Check sheet for the drawn part. Datum: minimum x, y, z corner. Units: mm. A direction names the side the tool comes from. Round coordinates to 2 decimals unless told otherwise and drop trailing zeros. Write each loop counter-clockwise with the first axis right and the second up, starting at its lowest first coordinate (ties: lowest second). Pieces come first, ordered by that corner, then holes. Notation, with made-up numbers: (-11, -27.5) - (2, -27.5) arc R21 ccw to (2, 5.5) - close; hole circle Ø1 at (-35.5, -16). An arc over 180 degrees is marked (long way). Return JSON: item names as keys, results as strings. Group by question number.
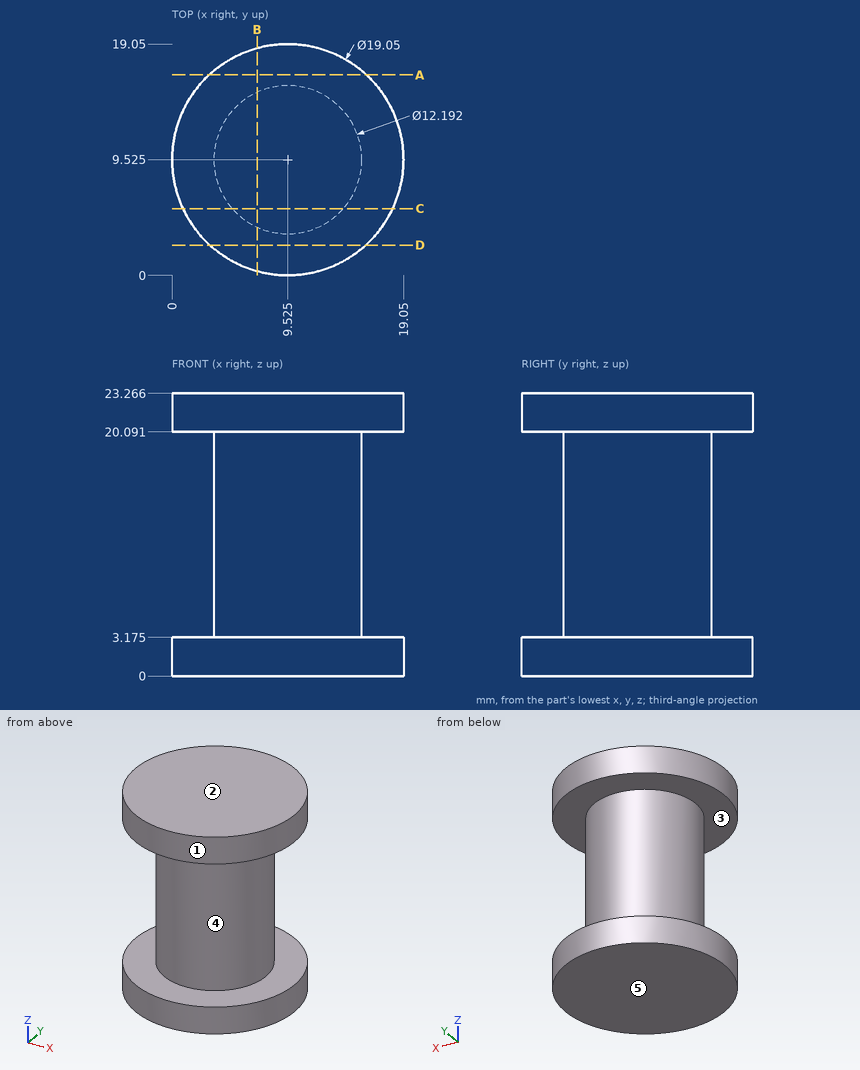
1. Mould release check, pull along Z, two halves, no side actions. Record for the marked faces 1, 2 and 3: pulls with the +Z half, pulls with the -Z half, needs draft (parallel to the pull), parting line crosses it, or undercut.
2. Material ranges on line 1 along Z through (x, y) = (3.5, 11.25) (1 decimal); line 2 along X through (y, z) = (9.75, 9.5); line 3 along Y through (x, z) = (5.25, 15.5), recorded low to high.
3. Section check B-B (x = 7). Enter the section's corners in (y, z) (1 decimal), and give its area (3 significant figures).
4. Tool access check on the marked faces 4 and 5. Record the directions out of +Z, -Z, +X, -X, +Y, -Y that give a thin tool (end or side, any length) a straight path to the whole face; none if there is none.
5. Section check C-C (y = 5.5). Enter the section's corners in (x, z) (1 decimal).
6. Section check D-D (y = 2.5). Enter the section's corners in (x, z) (1 decimal).
7. Section check A-A (y = 16.5). Enter the section's corners in (x, z) (1 decimal).
8. Depth check by flat-ended pin: pin 1 Ø2 at (y, z) = (6.5, 15) entering from -X (1 decimal); pin 2 Ø10 at (y, z) = (17, 19.5) entering from -X; pin 3 Ø8 at (x, z) = (8.5, 12) entering from -Y. Enter the tip coordinate at first touch or a pass-through.
Result sheet:
{
 "1": {"face 1": "needs draft", "face 2": "pulls with the +Z half", "face 3": "undercut"},
 "2": {"line 1": "z = 0 to 3.2, 20.1 to 23.3", "line 2": "x = 3.43 to 15.62", "line 3": "y = 5.18 to 13.87"},
 "3": {"outline": "(0.3, 0) - (18.7, 0) - (18.7, 3.2) - (15.1, 3.2) - (15.1, 20.1) - (18.7, 20.1) - (18.7, 23.3) - (0.3, 23.3) - (0.3, 20.1) - (4, 20.1) - (4, 3.2) - (0.3, 3.2) - close", "area": "304 mm²"},
 "4": {"face 4": "none", "face 5": "-Z, +X, -X, +Y, -Y"},
 "5": {"outline": "(0.9, 0) - (18.2, 0) - (18.2, 3.2) - (14.1, 3.2) - (14.1, 20.1) - (18.2, 20.1) - (18.2, 23.3) - (0.9, 23.3) - (0.9, 20.1) - (4.9, 20.1) - (4.9, 3.2) - (0.9, 3.2) - close"},
 "6": {"outline": "(3.1, 0) - (16, 0) - (16, 3.2) - (3.1, 3.2) - close; (3.1, 20.1) - (16, 20.1) - (16, 23.3) - (3.1, 23.3) - close"},
 "7": {"outline": "(3, 0) - (16, 0) - (16, 3.2) - (3, 3.2) - close; (3, 20.1) - (16, 20.1) - (16, 23.3) - (3, 23.3) - close"},
 "8": {"pin 1": "stops at x = 3.8", "pin 2": "stops at x = 0.34", "pin 3": "stops at y = 3.43"}
}
